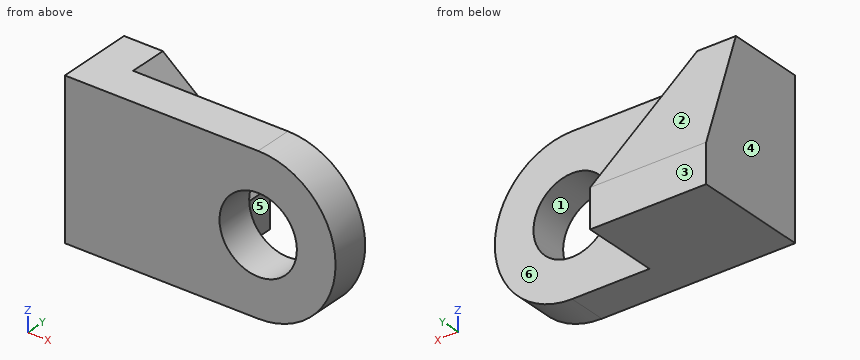
Autodesk Inventor part; units mm, degrees
ref_plane "YZ Plane" through (0, 0, 0) normal (1, 0, 0) x (0, 1, 0)
ref_plane "XZ Plane" through (0, 0, 0) normal (0, 1, 0) x (-1, 0, 0)
ref_plane "XY Plane" through (0, 0, 0) normal (0, 0, 1) x (1, 0, 0)
sketch "草圖1" plane through (0, 0, 0) normal (0, 1, 0) x (-1, 0, 0)
  circle A0 centre (0, 0) radius 20
  line L0 (0, -20) -> (50, -20)
  line L1 (50, -20) -> (50, 20)
  line L2 (50, 20) -> (0, 20)
  line L3 (0, 20) -> (0, -20)
  point P0 (0, 20)
  dimension "d0" = 40
  dimension "d1" = 50
extrude "擠出1" add sketch "草圖1" along normal blind 10
sketch "草圖2" plane through (0, 10, 0) normal (0, 1, 0) x (1, 0, 0)
  line L0 (-50, -20) -> (-50, 20)
  line L1 (-50, 20) -> (0, 20)
  arc A0 (0, -20) -> (0, 20) centre (0, 0) ccw
  line L2 (0, -20) -> (-50, -20)
  line L3 (-50, -20) -> (-50, 20)
  line L4 (-50, 20) -> (0, 20)
  arc A1 (0, -20) -> (0, 20) centre (0, 0) ccw
  line L5 (0, -20) -> (-50, -20)
  line L6 (0, 20) -> (-50, 20)
  line L7 (-50, 20) -> (-20, 20)
  line L8 (-20, 20) -> (-20, -20)
  line L9 (-20, -20) -> (-50, -20)
  line L10 (-50, -20) -> (-50, 20)
  line L11 (-50, -20) -> (0, -20)
  point P0 (-20, -20)
  point P1 (-20, 20)
  dimension "d4" = 30
extrude "擠出2" add sketch "草圖2" along normal blind 20 contours L0 L1 L8 L2
sketch "草圖3" plane through (0, 30, 0) normal (0, 1, 0) x (1, 0, 0)
  line L0 (-50, -20) -> (-50, 20)
  line L1 (-50, 20) -> (-20, 20)
  line L2 (-20, 20) -> (-20, -20)
  line L3 (-20, -20) -> (-50, -20)
  line L4 (-20, 10) -> (-40, -20)
  point P0 (0, 0)
  dimension "d7" = 10
  dimension "d8" = 10
extrude "擠出3" cut sketch "草圖3" against normal up to surface (20 mm away) contours L4 L2 L3
sketch "草圖6" plane through (-20, 10, -20) normal (1, 0, 0) x (0, 0, -1)
  line L0 (-10, 0) -> (-10, 20)
  line L1 (-10, 20) -> (0, 20)
  line L2 (0, 20) -> (0, 0)
  line L3 (-10, 0) -> (0, 0)
  line L4 (-40, 0) -> (-10, 0)
  line L5 (-40, -10) -> (-40, 0)
  line L6 (0, -10) -> (-40, -10)
  line L7 (0, 0) -> (0, -10)
  line L8 (-10, 20) -> (-10, 0)
  line L9 (-10, 20) -> (-40, 10)
  line L10 (-40, 10) -> (-10, 10)
  line L11 (-10, 10) -> (-10, 20)
  line L12 (-40, 0) -> (-40, 20)
  line L13 (-40, 20) -> (-10, 20)
  point P0 (-20, -10)
  dimension "d14" = 10
extrude "擠出4" cut sketch "草圖6" against normal blind 85.25 contours L9 L12 L13
sketch "草圖7" plane through (0, 10, 0) normal (0, 1, 0) x (1, 0, 0)
  arc A0 (0, -20) -> (0, 20) centre (0, 0) ccw
hole "孔1" at (0, 10, 0) direction (0, -1, 0) diameter 20 end through all
properties part number "27" material "鋼、碳鋼"
Verification items for the finished model (mm, model axes). Face numbers are marked on the shaded views. A direction names the side the tool comes from. Coordinates: 2 decimals unless noted, no trailing zeros. Order: outer loops, then holes, each group sorted by start corner. A loop starts at its lowest first (then second) coordinate and runs counter-clockwise, first axis right, second up. Notation, with made-up numbers: (17, 34) -> (48, 34) arc R19 cw to (48, 54) -> close; hole circle Ø11 at (36.5, -32.75). An arc over 180 degrees is marked (long way). Answer as CSV lines item,"result". Start each with the question number.
1) Material ranges on L1, parallel to Z at x = 0, y = 2.75; L2, parallel to X at y = 7.75, z = 0; L3, parallel to Y at x = -9, z = 14.5, recorded low to high. Write a range as [from, to].
2) Release check for a two-part mould opening along Z. For the marked faces 1, 2 and 3 record: released by +Z, released by -Z, zero draft, split by the parting line, or undercut.
3) Cross-section at D-D, the plane x = 5.5. Record the boundary of the cut face in (y, z), then the cut area to 3 significant figures.
4) Set-up check for the marked faces 4, 5 and 6: record each of +Z, -Z, +X, -X, +Y, -Y from which the full face is reachable in a straight line by a thin tool's end or side.
5) Cross-section at A-A, the plane z = 6. Record the boundary of the cut face in (x, y), then the cut area to 3 significant figures.
6) Cross-section at B-B, the plane x = -31. Record the boundary of the cut face in (y, z), then the cut area to 3 significant figures.
7) Gauge pin test, flat ends, axial feed: pin 1 Ø3 at (y, z) = (16, -15.5) entering from +X; pin 2 Ø3 at (x, z) = (-2, 14) entering from +Y; pin 3 Ø8 at (x, z) = (-39.5, -1) entering from +Y; pin 4 Ø16 at (x, z) = (0, 0) entering from +Y. Record the tip position at first contact, or that the pin passes through.
8) Cross-section at C-C, the plane y = 9. Record the boundary of the cut face in (x, z).
Conclusion:
1,L1,"z = [-20, -10], [10, 20]"
1,L2,"x = [-50, -10], [10, 20]"
1,L3,"y = [0, 10]"
2,face 1,"undercut"
2,face 2,"released by +Z"
2,face 3,"zero draft"
3,outline,"(0, -19.23) -> (10, -19.23) -> (10, -8.35) -> (0, -8.35) -> close; (0, 8.35) -> (10, 8.35) -> (10, 19.23) -> (0, 19.23) -> close"
3,area,"218 mm²"
4,face 4,"+Z, -Z, -X, +Y, -Y"
4,face 5,"+Z, -Z, +X, +Y"
4,face 6,"+Z, +X, +Y"
5,outline,"(-50, 0) -> (-8, 0) -> (-8, 10) -> (-30.67, 10) -> (-30.67, 24.67) -> (-50, 24.67) -> close; (8, 0) -> (19.08, 0) -> (19.08, 10) -> (8, 10) -> close"
5,area,"814 mm²"
6,outline,"(0, -20) -> (30, -20) -> (30, -10) -> (24.5, 6.5) -> (10, 6.5) -> (10, 20) -> (0, 20) -> close"
6,area,"885 mm²"
7,pin 1,"stops at x = -20"
7,pin 2,"stops at y = 10"
7,pin 3,"stops at y = 28.33"
7,pin 4,"passes through"
8,outline,"(-50, -20) -> (0, -20) arc R20 ccw to (0, 20) -> (-50, 20) -> close; hole circle Ø20 at (0, 0)"
